Geometry: final body of the model. Coordinates: model frame, mm. Face numbers are marked on the shaded views. A direction names the side the tool comes from. Give positions to 0.01 mm unless a question says otherwise; leave off trailing zeros. Loops run counter-clockwise (first coordinate to the right, second up) from the corner with the lowest first, then second, coordinate; pieces in that order, holes last. Notation, with made-up numbers: (76.5, 20.5) - (118.5, 20.5) arc R9 cw to (118.5, 26.5) - close; hole circle Ø1 at (1, -17.5). An arc over 180 degrees is marked (long way). Use one line per item in the form item = value.
```python
from build123d import *

# Parameters (mm, degrees)
BOSS_EXTRUDE1_DEPTH      = 6.55
BOSS_EXTRUDE1_DEPTH_BACK = 6.55
SKETCH2_W                = 12.5
SKETCH2_H                = 5.2
SKETCH2_W_2              = 10.75
SKETCH2_H_2              = 1.75
CUT_EXTRUDE1_DEPTH       = 9.5
BOSS_EXTRUDE2_DEPTH      = 0.3


with BuildPart() as part:
    # Sketch1 → Boss-Extrude1 (new body, two sides)
    with BuildSketch(Plane(origin=(0, 0, 0), x_dir=(0, 0, -1), z_dir=(1, 0, 0))) as boss_extrude1_sk:
        Polygon((-10.5, 10.35), (6.6, 10.35), (6.6, 0), (0, 0), (0, -5.27), (-10.5, -5.27), align=None)
    extrude(amount=BOSS_EXTRUDE1_DEPTH)
    extrude(boss_extrude1_sk.sketch, amount=-BOSS_EXTRUDE1_DEPTH_BACK)

    # Sketch2 → Cut-Extrude1 (cut)
    with BuildSketch(Plane.XY.offset(10.5)):
        with Locations((0, 6.75)):
            Rectangle(SKETCH2_W, SKETCH2_H)
        with Locations((0, 7.525)):
            Rectangle(SKETCH2_W_2, SKETCH2_H_2, mode=Mode.SUBTRACT)
        with Locations((0, -1.67)):
            Rectangle(SKETCH2_W, SKETCH2_H)
        with Locations((0, -0.895)):
            Rectangle(SKETCH2_W_2, SKETCH2_H_2, mode=Mode.SUBTRACT)
    extrude(amount=-CUT_EXTRUDE1_DEPTH, mode=Mode.SUBTRACT)

    # Sketch3 → Boss-Extrude2 (add)
    with BuildSketch(Plane(origin=(6.55, 0, 0), x_dir=(0, 0, -1), z_dir=(1, 0, 0))):
        with BuildLine():
            Line((3.6, -2.8), (3.075, -2.275))
            Line((3.075, -2.275), (3.075, -1.8))
            Line((3.075, -1.8), (3.3, -1.8))
            Line((3.3, -1.8), (3.3, 0))
            Line((3.3, 0), (4.3, 0))
            Line((4.3, 0), (4.3, -1.8))
            Line((4.3, -1.8), (4.525, -1.8))
            Line((4.525, -1.8), (4.525, -2.275))
            Line((4.525, -2.275), (4, -2.8))
            Line((4, -2.8), (4, -0.395))
            ThreePointArc((4, -0.395), (3.942885822, -0.257114178), (3.805, -0.2))
            Line((3.805, -0.2), (3.795, -0.2))
            ThreePointArc((3.795, -0.2), (3.657114178, -0.257114178), (3.6, -0.395))
            Line((3.6, -0.395), (3.6, -2.8))
        make_face()
    boss_extrude2 = extrude(amount=-BOSS_EXTRUDE2_DEPTH)

    # Mirror1: Boss-Extrude2 across plane
    add(boss_extrude2.mirror(Plane(origin=(0, 0, 0), x_dir=(0, 0, 1), z_dir=(1, 0, 0))))


solid = part.part
```
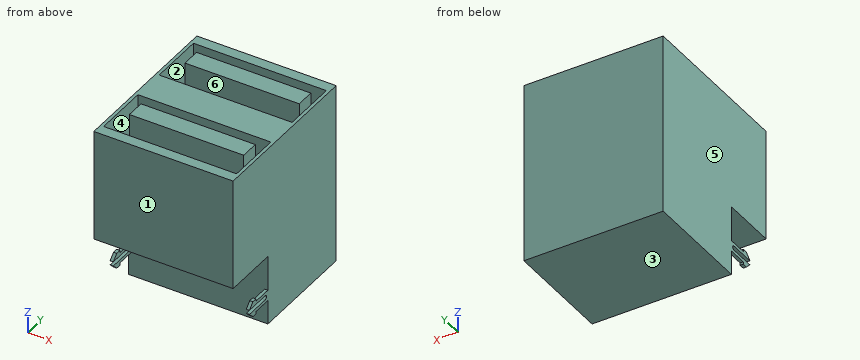
(1) Access query for the marked faces 5 and 6. Directions: +Z, -Z, +X, -X, +Y, -Y. A direction counts if a zero-diameter tool reaches every point of the face in a straight line with its end or side. Return the directions, or none.
Solution:
face_5 = +Z, -Z, -X, +Y, -Y
face_6 = +Z
(2) Pin query (flat end, axial travel): P1, Ø1.6, axis at x = -1.5, y = 6, coming from the +Z side. Return the tip coordinate at first contact, or that it passes through.
Solution:
P1 = 10.5
(3) Pull-direction query (Y, two-part tool) for the marked faces 1, 2, 3 and 4; classes: released by +Y, released by -Y, zero draft, split by the parting line, or undercut.
Solution:
face_1 = released by -Y
face_2 = undercut
face_3 = zero draft
face_4 = undercut
(4) Material intervals for L1, parallel to Y at x = -3.5, z = 4.75; L2, parallel to X at y = 7.25, z = 3 (3 decimals); L3, parallel to Y at x = -5.5, z = 2.75, sorted ascending. Write a range as from..to.
Solution:
L1 = -5.27..-4.27, -1.77..-0.02, 0.93..4.15, 6.65..8.4, 9.35..10.35
L2 = -6.55..-6.25, -5.375..5.375, 6.25..6.55
L3 = -5.27..-4.27, 0.93..4.15, 9.35..10.35
(5) Cut plane A-A (z = 6.5). Return the cut outline in (x, y) (3 decimals), plus the area to 3 significant figures.
Solution:
outline = (-6.55, -5.27) - (6.55, -5.27) - (6.55, 10.35) - (-6.55, 10.35) - close; (-5.375, -1.77) - (5.375, -1.77) - (5.375, -0.02) - (-5.375, -0.02) - close; (-5.375, 6.65) - (5.375, 6.65) - (5.375, 8.4) - (-5.375, 8.4) - close; hole (-6.25, -4.27) - (6.25, -4.27) - (6.25, 0.93) - (-6.25, 0.93) - close; hole (-6.25, 4.15) - (6.25, 4.15) - (6.25, 9.35) - (-6.25, 9.35) - close
area = 112 mm2
(6) Cut plane B-B (y = -0.75). Return the cut outline in (x, z) (3 decimals), plus the area to 3 significant figures.
Solution:
outline = (-6.55, -4.3) - (-6.25, -4.3) - (-6.25, -4) - (-6.55, -4) - close; (-6.55, -3.6) - (-6.25, -3.6) - (-6.25, -3.3) - (-6.55, -3.3) - close; (-6.55, 0) - (6.55, 0) - (6.55, 10.5) - (6.25, 10.5) - (6.25, 1) - (5.375, 1) - (5.375, 10.5) - (-5.375, 10.5) - (-5.375, 1) - (-6.25, 1) - (-6.25, 10.5) - (-6.55, 10.5) - close; (6.25, -4.3) - (6.55, -4.3) - (6.55, -4) - (6.25, -4) - close; (6.25, -3.6) - (6.55, -3.6) - (6.55, -3.3) - (6.25, -3.3) - close
area = 121 mm2
(7) Cut plane D-D (z = -1). Return the cut outline in (x, y), plus the area to 3 significant figures.
Solution:
outline = (-6.55, 0) - (6.55, 0) - (6.55, 10.35) - (-6.55, 10.35) - close
area = 136 mm2
(8) Cut plane C-C (x = -1.75). Return the cut outline in (y, z), plus the area to 3 significant figures.
Solution:
outline = (-5.27, 0) - (0, 0) - (0, -6.6) - (10.35, -6.6) - (10.35, 10.5) - (9.35, 10.5) - (9.35, 1) - (8.4, 1) - (8.4, 10.5) - (6.65, 10.5) - (6.65, 1) - (4.15, 1) - (4.15, 10.5) - (0.93, 10.5) - (0.93, 1) - (-0.02, 1) - (-0.02, 10.5) - (-1.77, 10.5) - (-1.77, 1) - (-4.27, 1) - (-4.27, 10.5) - (-5.27, 10.5) - close
area = 167 mm2
